```python
from build123d import *

# Parameters (mm, degrees)
F1_DEPTH = 1524
F2_SIZE  = 1.27
F3_SIZE  = 1.27
F5_DEPTH = 152.4


with BuildPart() as f1:
    # F0 (on Right) → F1 (new body)
    with BuildSketch(Plane.YZ):
        Polygon((101.6, 101.6), (-101.6, 101.6), (-101.6, 94.361), (-3.6195, 94.361), (-3.6195, 0), (0, 0), (3.6195, 0), (3.6195, 94.361), (101.6, 94.361), align=None)
        Polygon((0, 0), (-3.6195, 0), (-3.6195, -94.361), (-101.6, -94.361), (-101.6, -101.6), (101.6, -101.6), (101.6, -94.361), (3.6195, -94.361), (3.6195, 0), align=None)
    extrude(amount=F1_DEPTH)

    # F2
    f2_edges = [f1.edges().sort_by_distance(p)[0] for p in [
        (762, -101.6, 101.6),
        (762, -101.6, 94.361),
        (762, 101.6, 101.6),
        (762, 101.6, 94.361),
        (762, 101.6, -94.361),
        (762, 101.6, -101.6),
        (762, -101.6, -94.361),
        (762, -101.6, -101.6),
    ]]
    chamfer(f2_edges, length=F2_SIZE)

    # F3
    f3_edges = [f1.edges().sort_by_distance(p)[0] for p in [
        (762, -3.6195, 94.361),
        (762, 3.6195, 94.361),
        (762, 3.6195, -94.361),
        (762, -3.6195, -94.361),
    ]]
    chamfer(f3_edges, length=F3_SIZE)

    # F4 (on face) → F5 (join)
    with BuildSketch(Plane.XY.offset(101.6)):
        Polygon((152.4, 12.7), (152.4, -12.7), (254, -12.7), (266.7, 0), (254, 12.7), align=None)
    extrude(amount=F5_DEPTH)


solid = f1.part
```
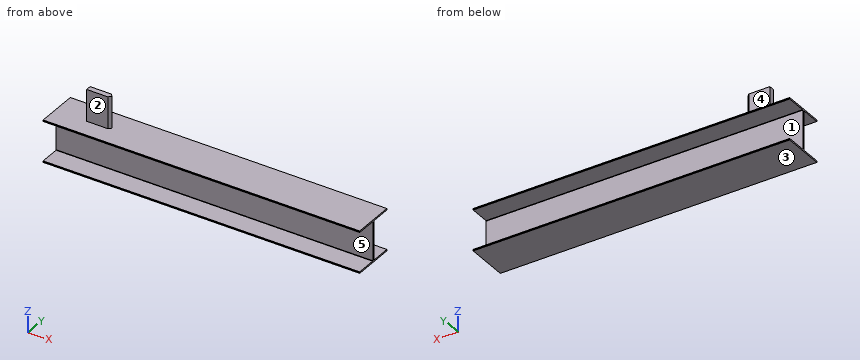
Source: CAD feature listing. Evaluate the final solid. Frame: model axes, mm. Face numbers are marked on the shaded views. A direction names the side the tool comes from. Give positions to 0.01 mm unless a question says otherwise; leave off trailing zeros. Loops run counter-clockwise (first coordinate to the right, second up) from the corner with the lowest first, then second, coordinate; pieces in that order, holes last. Notation, with made-up numbers: (-2.75, 61) -> (41.25, 61) arc R27 cw to (41.25, 90) -> close; hole circle Ø4 at (2.5, 56). An arc over 180 degrees is marked (long way). Use a Markdown table: item, result. Add a question column.
(1) Section query A-A (y = -64). Output: boundary loops of the cut face in (x, z).
(2) Ray query, line 1 (Z direction, x = 105.5, y = -90); line 2 (Y direction, x = 414.5, z = 38); line 3 (Y direction, x = 171.5, z = 101.5). Return the intervals inside material, ascending.
(3) Section query B-B (z = 120.5). Output: boundary loops of the cut face in (x, y), then the cut area to 3 significant figures.
(4) Section query D-D (z = 61). Output: boundary loops of the cut face in (x, y), then the cut area to 3 significant figures.
(5) Section query C-C (x = 573.5). Output: boundary loops of the cut face in (y, z).
(6) Access query for the marked faces 4 and 5. Directions: +Z, -Z, +X, -X, +Y, -Y. A direction counts if a zero-diameter tool reaches every point of the face in a straight line with its end or side. Return the directions, or none.
(7) Pull-direction query (Z, two-part tool) for the marked faces 1, 2 and 3; classes: +Z half, -Z half, draft (parallel to the pull), parting line (faces both ways), or undercut.
(8) First-contact query: pin 1 Ø8 at (x, z) = (506.5, 32) entering from +Y; pin 2 Ø6 at (x, y) = (715.5, 57) entering from +Z; pin 3 Ø1 at (x, z) = (530.5, -21.5) entering from -Y; pin 4 Ø5 at (x, z) = (728.5, 93.5) entering from +Y. Flat tips, straight axial feed; report the tip coordinate or a pass-through.
Checked values:
| question | item | result |
|---|---|---|
| 1 | outline | (0, -101.6) -> (1524, -101.6) -> (1524, -94.36) -> (0, -94.36) -> close; (0, 94.36) -> (1524, 94.36) -> (1524, 101.6) -> (0, 101.6) -> close |
| 2 | line 1 | -101.6 to -94.36, 94.36 to 101.6 |
| 2 | line 2 | -3.62 to 3.62 |
| 2 | line 3 | -100.43 to 100.43 |
| 3 | outline | (152.4, -12.7) -> (254, -12.7) -> (266.7, 0) -> (254, 12.7) -> (152.4, 12.7) -> close |
| 3 | area | 2,740 mm^2 |
| 4 | outline | (0, -3.62) -> (1524, -3.62) -> (1524, 3.62) -> (0, 3.62) -> close |
| 4 | area | 11,000 mm^2 |
| 5 | outline | (-101.6, -100.33) -> (-100.33, -101.6) -> (100.33, -101.6) -> (101.6, -100.33) -> (101.6, -95.63) -> (100.33, -94.36) -> (4.89, -94.36) -> (3.62, -93.09) -> (3.62, 93.09) -> (4.89, 94.36) -> (100.33, 94.36) -> (101.6, 95.63) -> (101.6, 100.33) -> (100.33, 101.6) -> (-100.33, 101.6) -> (-101.6, 100.33) -> (-101.6, 95.63) -> (-100.33, 94.36) -> (-4.89, 94.36) -> (-3.62, 93.09) -> (-3.62, -93.09) -> (-4.89, -94.36) -> (-100.33, -94.36) -> (-101.6, -95.63) -> close |
| 6 | face 4 | +Z, +X, -X, +Y |
| 6 | face 5 | +X, -X, -Y |
| 7 | face 1 | undercut |
| 7 | face 2 | draft |
| 7 | face 3 | -Z half |
| 8 | pin 1 | y = 3.62 |
| 8 | pin 2 | z = 101.6 |
| 8 | pin 3 | y = -3.62 |
| 8 | pin 4 | y = 101.6 |
